Design review of the part built by this model. Coordinates are the model's own, in mm. A direction names the side the tool comes from. Coordinates: 2 decimals unless noted, no trailing zeros. Write each loop counter-clockwise with the first axis right and the second up, starting at its lowest first coordinate (ties: lowest second). Pieces come first, ordered by that corner, then holes.
Autodesk Inventor part; units mm, degrees
ref_plane "YZ Plane" through (0, 0, 0) normal (1, 0, 0) x (0, 1, 0)
ref_plane "XZ Plane" through (0, 0, 0) normal (0, 1, 0) x (-1, 0, 0)
ref_plane "XY Plane" through (0, 0, 0) normal (0, 0, 1) x (1, 0, 0)
sketch "Skizze2" plane through (0, 0, 0) normal (0, 1, 0) x (-1, 0, 0)
  circle A0 centre (0, 0) radius 30
  dimension "d3" = 60
extrude "Extrusion2" add sketch "Skizze2" along normal blind 5
sketch "Skizze3" plane through (0, 5, 0) normal (0, 1, 0) x (1, 0, 0)
  circle A0 centre (0, 0) radius 10.5
  dimension "d6" = 21
extrude "Extrusion3" add sketch "Skizze3" along normal blind 7
sketch "Skizze4" plane through (0, 0, 0) normal (0, -1, 0) x (1, 0, 0)
  circle A0 centre (0, 0) radius 7.5
  dimension "d9" = 15
extrude "Extrusion4" add sketch "Skizze4" along normal blind 10
sketch "Skizze5" plane through (0, -10, 0) normal (0, -1, 0) x (1, 0, 0)
  arc A0 (1.5166, -2.05) -> (-1.5166, -2.05) centre (0, 0) ccw
  line L0 (1.5166, -2.05) -> (-1.5166, -2.05)
  dimension "d12" = 5.1
  dimension "d14" = 4.6
extrude "Extrusion5" cut sketch "Skizze5" against normal blind 20
sketch "Skizze6" plane through (-1.5166, -10, -2.05) normal (0, 0, 1) x (1, 0, 0)
  line L0 (-5.9834, 0) -> (9.0166, 0)
  line L1 (1.5166, 0) -> (1.5166, 10)
  line L2 (1.5166, 10) -> (1.5166, 0)
  circle A0 centre (1.5166, 5) radius 1
  dimension "d17" = 2
  dimension "d20" = 5
extrude "Extrusion6" cut sketch "Skizze6" against normal blind 20
sketch "Skizze7" plane through (0, -10, 0) normal (0, -1, 0) x (1, 0, 0)
  circle A0 centre (0, 0) radius 7.5
  line L0 (2.6926, -7) -> (-2.6926, -7)
  point P0 (0, -7)
  dimension "d23" = 7
extrude "Extrusion7" cut sketch "Skizze7" against normal blind 10 contours L0 A0 picked at (0.3052, -7.148)
sketch "Skizze8" plane through (0, 0, 0) normal (0, -1, 0) x (1, 0, 0)
  circle A0 centre (0, 0) radius 24 construction
  line L0 (20.7846, 12) -> (20.7846, -12) construction
  line L1 (20.7846, -12) -> (0, -24) construction
  line L2 (0, -24) -> (-20.7846, -12) construction
  line L3 (-20.7846, -12) -> (-20.7846, 12) construction
  line L4 (-20.7846, 12) -> (0, 24) construction
  line L5 (0, 24) -> (20.7846, 12) construction
  circle A1 centre (0, 0) radius 30
  line L6 (30, 0) -> (-30, 0)
  line L7 (0, -30) -> (0, 30)
  circle A2 centre (0, -24) radius 2
  circle A3 centre (20.7846, -12) radius 2
  circle A4 centre (20.7846, 12) radius 2
  circle A5 centre (0, 24) radius 2
  circle A6 centre (-20.7846, 12) radius 2
  circle A7 centre (-20.7846, -12) radius 2
  dimension "d26" = 48
  dimension "d27" = 24
  dimension "d28" = 4
  dimension "d29" = 4
  dimension "d30" = 4
  dimension "d31" = 4
  dimension "d32" = 4
  dimension "d33" = 4
extrude "Extrusion8" cut sketch "Skizze8" against normal blind 20 contours A5 L7 | L7 A5 | A2 L7 | L7 A2 | A3 | A4 | A6 | A7
sketch "Skizze9" plane through (0, 12, 0) normal (0, 1, 0) x (1, 0, 0)
  arc A0 (-1.5166, 2.05) -> (1.5166, 2.05) centre (0, 0) ccw
  circle A1 centre (0, 0) radius 8.5
  dimension "d36" = 17
extrude "Extrusion9" add sketch "Skizze9" along normal blind 7.5
sketch "Skizze11" plane through (0, 19.5, 0) normal (0, 1, 0) x (1, 0, 0)
  circle A0 centre (0, 0) radius 2
  dimension "d47" = 4
extrude "Extrusion10" cut sketch "Skizze11" against normal blind 50
properties part number "Radaufhängung_06"
(1) Mouldability with a two-part tool opening along Z and no side actions: class faces 6 (the cylindrical face through (4.57, 15.698, 7.167)), 7 (the flat face through (-2, -10, 2)), 8 (the cylindrical face through (0.923, 2.465, 22.226)) as +Z half, -Z half, draft (parallel to the pull), parting line (faces both ways), or undercut.
(2) For faces 1 (the flat face through (0, 0, -2.05)), 2 (the cylindrical face through (0, -4, -4)), 3 (the cylindrical face through (18.787, 2.465, 12.088)), 4 (the flat face through (-13, 5, 0)), 5 (the flat face through (0, -6.2, -7)), list the 3-axis set-ups (+Z, -Z, +X, -X, +Y, -Y) from which the entire face can be reached by the end or side of a thin tool; tool diameter is ignored.
(3) Consider section D-D (z = -5). Give the boundary of the cut face in (x, y).
(4) Consider section C-C (y = -5). Give the boundary of the cut face in (x, z), plus the area to 3 significant figures.
(5) Insertion check: pin 1 Ø3.5 at (x, y) = (0.5, 0) entering from +Z; pin 2 Ø2 at (x, z) = (-13, 17) entering from +Y; pin 3 Ø1 at (x, z) = (4, 9) entering from +Y. Each pin has a flat end and moves straight along its axis. Give the tip position at first contact, or say it passes through.
(6) Consider section B-B (x = 21.5). Give the boundary of the cut face in (y, z), plus the area to 3 significant figures.
(7) Consider section A-A (z = -24). Give the boundary of the cut face in (x, y).
(8) Wall thickness on line 1 (Z direction, x = 0, y = 2.25); line 2 (Z direction, x = 0, y = 13.5); line 3 (X direction, y = 2.25, z = 11.5): over which ranges is each line inside the solid? List them lowest first.
Results:
1. face 6: parting line
1. face 7: draft
1. face 8: undercut
2. face 1: -Y
2. face 2: -Z
2. face 3: +Y, -Y
2. face 4: +Y
2. face 5: -Z, +X, -X, -Y
3. outline: (-29.58, 0) - (-5.59, 0) - (-5.59, -10) - (5.59, -10) - (5.59, 0) - (29.58, 0) - (29.58, 5) - (9.23, 5) - (9.23, 12) - (6.87, 12) - (6.87, 19.5) - (-6.87, 19.5) - (-6.87, 12) - (-9.23, 12) - (-9.23, 5) - (-29.58, 5) - close; hole circle Ø2 at (0, -5)
4. outline: (-2.69, -7) - (-1, -7) - (-1, -2.05) - (-1.52, -2.05) arc R2.55 cw (long way) to (1.52, -2.05) - (1, -2.05) - (1, -7) - (2.69, -7) arc R7.5 ccw (long way) to start
4. area: 146 mm2
5. pin 1: stops at z = 30
5. pin 2: stops at y = 5
5. pin 3: stops at y = 12
6. outline: (0, -20.92) - (5, -20.92) - (5, -13.87) - (0, -13.87) - close; (0, -10.13) - (5, -10.13) - (5, 10.13) - (0, 10.13) - close; (0, 13.87) - (5, 13.87) - (5, 20.92) - (0, 20.92) - close
6. area: 172 mm2
7. outline: (-18, 0) - (-2, 0) - (-2, 5) - (-18, 5) - close; (2, 0) - (18, 0) - (18, 5) - (2, 5) - close
8. line 1: z = -30 to -26, -22 to -2.05, 2.55 to 22, 26 to 30
8. line 2: z = -8.5 to -2, 2 to 8.5
8. line 3: x = -27.71 to -22.72, -18.85 to 18.85, 22.72 to 27.71
